Design review of the part built by this model. Coordinates are the model's own, in mm. A direction names the side the tool comes from. Coordinates: 2 decimals unless noted, no trailing zeros. Loops run counter-clockwise (first coordinate to the right, second up) from the corner with the lowest first, then second, coordinate; pieces in that order, holes last. Notation, with made-up numbers: (38, -4) -> (79, -4) arc R19 ccw to (79, 3) -> close; hole circle Ø6 at (66, 16.25). An arc over 180 degrees is marked (long way). Use CSV: the item, a comma, the result in double quotes.
```python
from build123d import *

# Parameters (mm, degrees)
F1_DEPTH = 25.4
F3_D     = 15.24


with BuildPart() as f1:
    # F0 (on Front) → F1 (new body)
    with BuildSketch(Plane.XZ):
        Polygon((-31.079613, 5.679613), (-25.999613, 0), (-20.32, 5.08), (0, 5.08), (20.32, 5.08), (25.999613, 0), (31.079613, 5.679613), (25.4, 10.759613), (0, 10.759613), (-25.4, 10.759613), align=None)
    extrude(amount=F1_DEPTH)

    # F3 (through all)
    with Locations(Plane.XY.offset(10.759613)):
        with Locations((0, -12.7)):
            Hole(F3_D / 2)


solid = f1.part
```
Item 1: Machinability: for faces 1 (the face through (23.12, -12.522, 2.576)), 2 (the face through (28.504, -12.522, 2.8)), which of the approach directions +Z, -Z, +X, -X, +Y, -Y give a long, thin tool a straight path to every point of the face, cutting with its end or side? Answer none if there is none.
Checked values:
face 1,"-Z, +Y, -Y"
face 2,"-Z, +X, +Y, -Y"
Item 2: Add section C-C (y = -22). Give the boundary of the cut face in (x, z), then the cut area to 3 significant figures.
Checked values:
outline,"(-31.08, 5.68) -> (-26, 0) -> (-20.32, 5.08) -> (20.32, 5.08) -> (26, 0) -> (31.08, 5.68) -> (25.4, 10.76) -> (-25.4, 10.76) -> close"
area,"376 mm^2"
Item 3: To check wall thickness, follow line 1 along Y through (x, z) = (0, 8.9); line 2 along Z through (x, y) = (-15, -14.25); line 3 along X through (y, z) = (-8.25, 4). State the ranges of each line that lie inside material, in increasing order.
Checked values:
line 1,"-25.4 to -20.32, -5.08 to 0"
line 2,"5.08 to 10.76"
line 3,"-29.58 to -21.53, 21.53 to 29.58"
Item 4: Clearance check with flat-ended pins moving along their axes: pin 1 (5 mm diameter, centred on y = -5.5, z = 8, fed in from +X); pin 2 (5 mm diameter, centred on x = 17, y = -13.5, fed in from -Z); pin 3 (13.5 mm diameter, centred on x = 0, y = -12.7, fed in from -Z). State where each tip first meets the part, or that it passes through.
Checked values:
pin 1,"x = 31.08"
pin 2,"z = 5.08"
pin 3,"through"
Item 5: Add section B-B (y = -12.7). Give the boundary of the cut face in (x, z).
Checked values:
outline,"(-31.08, 5.68) -> (-26, 0) -> (-20.32, 5.08) -> (-7.62, 5.08) -> (-7.62, 10.76) -> (-25.4, 10.76) -> close; (7.62, 5.08) -> (20.32, 5.08) -> (26, 0) -> (31.08, 5.68) -> (25.4, 10.76) -> (7.62, 10.76) -> close"
Item 6: Add section D-D (z = 1). Give the boundary of the cut face in (x, y).
Checked values:
outline,"(-26.89, -25.4) -> (-24.88, -25.4) -> (-24.88, 0) -> (-26.89, 0) -> close; (24.88, -25.4) -> (26.89, -25.4) -> (26.89, 0) -> (24.88, 0) -> close"
Item 7: Add section A-A (x = 0). Give the boundary of the cut face in (y, z), then the cut area to 3 significant figures.
Checked values:
outline,"(-25.4, 5.08) -> (-20.32, 5.08) -> (-20.32, 10.76) -> (-25.4, 10.76) -> close; (-5.08, 5.08) -> (0, 5.08) -> (0, 10.76) -> (-5.08, 10.76) -> close"
area,"57.7 mm^2"
